from build123d import *

# Parameters (mm, degrees)
F0_W     = 124
F0_H     = 80
F1_DEPTH = 7
F3_DEPTH = 25
F5_DEPTH = 25
F6_R     = 2.897056


with BuildPart() as f1:
    # F0 (on Top) → F1 (new body)
    with BuildSketch(Plane.XY):
        with Locations((-62, 40)):
            Rectangle(F0_W, F0_H)
    extrude(amount=F1_DEPTH)

    # F2 (on face) → F3 (cut)
    with BuildSketch(Plane.XY.offset(7)):
        with BuildLine():
            ThreePointArc((-25, 55), (-35.242641, 59.242641), (-31, 49))
            ThreePointArc((-31, 49), (-26.757359, 50.757359), (-25, 55))
        make_face()
        with BuildLine():
            ThreePointArc((-25, 25), (-26.757359, 29.242641), (-31, 31))
            ThreePointArc((-31, 31), (-35.242641, 20.757359), (-25, 25))
        make_face()
    extrude(amount=-F3_DEPTH, mode=Mode.SUBTRACT)

    # F4 (on face) → F5 (cut)
    with BuildSketch(Plane.XY.offset(7)):
        Polygon((-94, 55.5), (-94, 40), (-94, 24.5), (-87, 24.5), (-87, 55.5), align=None)
    extrude(amount=-F5_DEPTH, mode=Mode.SUBTRACT)

    # F6
    f6_edges = [f1.edges().sort_by_distance(p)[0] for p in [
        (-87, 55.5, 3.5),
        (-94, 55.5, 3.5),
        (-87, 24.5, 3.5),
        (-94, 24.5, 3.5),
    ]]
    fillet(f6_edges, radius=F6_R)


solid = f1.part
CAD build for the part. Positions are in the model's coordinates, mm. A direction names the side the tool comes from. Coordinates: 2 decimals unless noted, no trailing zeros. Order: outer loops, then holes, each group sorted by start corner. A loop starts at its lowest first (then second) coordinate and runs counter-clockwise, first axis right, second up.
Item 1: Pin check, flat tip, straight feed: pin 1 Ø9.5 at (x, y) = (-31, 25) entering from +Z. Stop position of the tip, or through.
Check sheet entries:
pin 1: passes through
Item 2: Band-saw the part on B-B on y = 57.5. List the corners of the cut face in (x, z).
Check sheet entries:
outline: (-124, 0) - (-36.45, 0) - (-36.45, 7) - (-124, 7) - close; (-25.55, 0) - (0, 0) - (0, 7) - (-25.55, 7) - close
Item 3: Band-saw the part on A-A on y = 36.5. List the corners of the cut face in (x, z).
Check sheet entries:
outline: (-124, 0) - (-94, 0) - (-94, 7) - (-124, 7) - close; (-87, 0) - (0, 0) - (0, 7) - (-87, 7) - close
Item 4: Drill centre lines: L1, parallel to Y at x = -31, z = 4; L2, parallel to X at y = 30, z = 3; L3, parallel to X at y = 55, z = 3.5. Where is each one in solid material? Low to high.
Check sheet entries:
L1: y = 0 to 19, 31 to 49, 61 to 80
L2: x = -124 to -94, -87 to -34.32, -27.68 to 0
L3: x = -124 to -92.73, -88.27 to -37, -25 to 0
Item 5: 3-axis set-ups, long thin cutter, end or side, ignore diameter. For faces 4 (the face through (-63, 0, 3)), 5 (the face through (-87, 40, 4)): which of +Z, -Z, +X, -X, +Y, -Y reach the whole face in a straight line?
Check sheet entries:
face 4: +Z, -Z, +X, -X, -Y
face 5: +Z, -Z
Item 6: Two-plate mould, pull along X, no slides. Class faces 1 (the face through (-63, 80, 3)), 2 (the face through (-87.9, 25.3, 3.5)), 3 (the face through (-124, 39, 3)): +X half, -X half, draft (parallel to the pull), parting line (faces both ways), or undercut.
Check sheet entries:
face 1: draft
face 2: undercut
face 3: -X half
